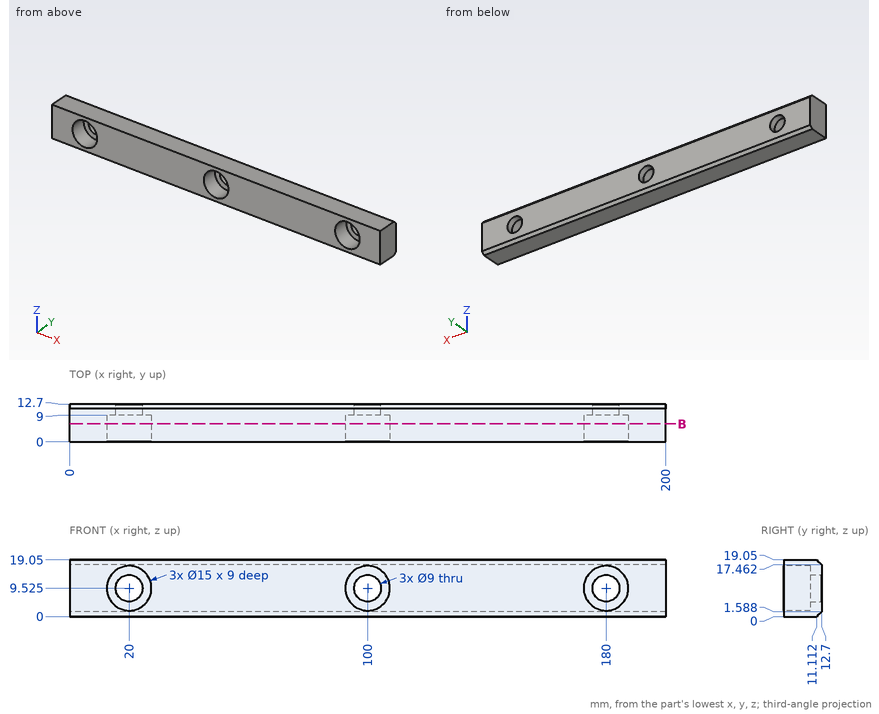
Geometry check sheet. Reference: drawing and pictorial views, mm from the part's lowest x, y, z. Coordinates: 2 decimals unless noted, no trailing zeros. Write item = value, one per line. Start each with the question number.
1. Thickness scan on probe 1 along X at (y, z) = (1, 15.5) (1 decimal); probe 2 along X at (y, z) = (4.25, 9.25) (1 decimal); probe 3 along Y at (x, z) = (93, 8.5). Record the ranges inside material, lowest first.
2. Go/stop test with flat-tipped pins: pin 1 (4.5 mm diameter, centred on x = 19, z = 13, fed in from -Y); pin 2 (7 mm diameter, centred on x = 20, z = 9.525, fed in from +Y). Record where each tip stops, or that it passes through.
3. Sectioned sample at B-B (y = 6). State how many separate pieces and enclosed holes the cut face has, then the cut area to 3 significant figures.
The answers:
q1.probe_1 = 0 to 15.5, 24.5 to 95.5, 104.5 to 175.5, 184.5 to 200
q1.probe_2 = 0 to 12.5, 27.5 to 92.5, 107.5 to 172.5, 187.5 to 200
q1.probe_3 = 9 to 12.7
q2.pin_1 = 9
q2.pin_2 = through
q3.separate_pieces = 1
q3.enclosed_holes = 3
q3.area = 3,280 mm²
